Can you work these out from the model? Positions are in its coordinate system, mm. A direction names the side the tool comes from. Coordinates: 2 decimals unless noted, no trailing zeros. Loops run counter-clockwise (first coordinate to the right, second up) from the corner with the lowest first, then second, coordinate; pieces in that order, holes last. Notation, with made-up numbers: M 15,82.25 L 53,82.25 A25 cw 53,119.25 Z; hole C -14.75,35.5 d2. An arc over 180 degrees is marked long. Answer as a JSON object with one key per item and string values. Group by question number.
Item 1: Which directions (+Z, -Z, +X, -X, +Y, -Y) give clear straight access to the entire face, cutting with the end or side of a thin tool? Please do faces 1 (the flat face through (36, 16, 67)), 2 (the flat face through (36, -13.82, 34)).
Item 2: Suppose I cut it at B-B (x = 11). Write out the boundary of the cut face in (y, z).
Item 3: Suppose I cut it at C-C (z = 38). Write out the boundary of the cut face in (x, y), then the cut area to 3 significant figures.
Item 4: Suppose I cut it at D-D (y = -5). Write out the boundary of the cut face in (x, z), then the cut area to 3 significant figures.
Item 5: If I drill on line 1 (Z direction, x = -54, y = 15.5); line 2 (X direction, y = 24.5, z = 38); line 3 (Y direction, x = 38, z = 21), over which ranges is the centre line in solid material (lowest first)?
Item 6: I'm going to push flat-ended pins straight in: pin 1 Ø0.6 at (x, z) = (-71.5, 18.5) entering from +Y; pin 2 Ø1 at (x, z) = (-39.5, 67.5) entering from +Y; pin 3 Ø1.6 at (x, z) = (112.5, 68) entering from +Y. Where does each tip first touch, or does it pass through?
Item 7: Suppose I cut it at A-A (y = 32.5). Write out the boundary of the cut face in (x, z).
Item 8: We'd pull the mould along Z, two halves only. Please class faces 3 (the flat face through (36, 16, 2)), 4 (the flat face through (68, 43.18, 1)), 5 (the flat face through (36, 15, 0)): +Z half, -Z half, draft (parallel to the pull), parting line (faces both ways), or undercut.
```python
from build123d import *

# Parameters (mm, degrees)
ESQUISSE1_W            = 220
ESQUISSE1_H            = 57
BOSS_EXTRU_1_DEPTH     = 69
COQUE1_T               = -2
ESQUISSE2_W            = 42.430934458
ESQUISSE2_H            = 23.81944652
TROU_CABLES_DEPTH      = 10
ESQUISSE4_W            = 39.063130892
ESQUISSE4_H            = 19.851704837
TROU_BORNIER_DEPTH     = 10
ESQUISSE5_W            = 15.700605502
ESQUISSE5_H            = 14.772120087
TROU_RASPBERRY_1_DEPTH = 10
ESQUISSE6_W            = 14.187422576
ESQUISSE6_H            = 17.21673515
TROU_RASPBERRY_2_DEPTH = 10
ESQUISSE7_W            = 14.101040577
ESQUISSE7_H            = 17.33071114
TROU_RASPBERRY_3_DEPTH = 10
ESQUISSE8_W            = 7.498357612
ESQUISSE8_H            = 7.301962728
TROU_RASPBERRY_4_DEPTH = 10
ESQUISSE9_W            = 15.051909722
ESQUISSE9_H            = 7.770311475
TROU_RASPBERRY_5_DEPTH = 10
ESQUISSE10_W           = 8.572607217
ESQUISSE10_H           = 3.212302761
TROU_RASPBERRY_6_DEPTH = 10


with BuildPart() as part:
    # Esquisse1 → Boss.-Extru.1 (new body)
    with BuildSketch(Plane.XY):
        with Locations((37.797752809, 14.679775281)):
            Rectangle(ESQUISSE1_W, ESQUISSE1_H)
    extrude(amount=BOSS_EXTRU_1_DEPTH)

    # Coque1
    coque1_openings = [part.faces().sort_by_distance(p)[0] for p in [
        (37.797752809, 43.179775281, 34.5),
    ]]
    offset(amount=COQUE1_T, openings=coque1_openings, kind=Kind.INTERSECTION)

    # Esquisse2 → Trou cables (cut)
    with BuildSketch(Plane(origin=(0, 0, 0), x_dir=(-1, 0, 0), z_dir=(0, 0, -1))):
        with Locations((45.673767677, 31.270052021)):
            Rectangle(ESQUISSE2_W, ESQUISSE2_H)
    extrude(amount=-TROU_CABLES_DEPTH, mode=Mode.SUBTRACT)

    # Esquisse4 → trou bornier (cut)
    with BuildSketch(Plane.XY.offset(69)):
        with Locations((116.674495492, 33.253922863)):
            Rectangle(ESQUISSE4_W, ESQUISSE4_H)
    extrude(amount=-TROU_BORNIER_DEPTH, mode=Mode.SUBTRACT)

    # Esquisse5 → trou raspberry 1 (cut)
    with BuildSketch(Plane.ZY.offset(72.202247191)):
        with Locations((56.756295127, 35.793715238)):
            Rectangle(ESQUISSE5_W, ESQUISSE5_H)
    extrude(amount=-TROU_RASPBERRY_1_DEPTH, mode=Mode.SUBTRACT)

    # Esquisse6 → trou raspberry 2 (cut)
    with BuildSketch(Plane.ZY.offset(72.202247191)):
        with Locations((37.961253625, 34.571407706)):
            Rectangle(ESQUISSE6_W, ESQUISSE6_H)
    extrude(amount=-TROU_RASPBERRY_2_DEPTH, mode=Mode.SUBTRACT)

    # Esquisse7 → trou raspberry 3 (cut)
    with BuildSketch(Plane.ZY.offset(72.202247191)):
        with Locations((19.999072944, 34.514419711)):
            Rectangle(ESQUISSE7_W, ESQUISSE7_H)
    extrude(amount=-TROU_RASPBERRY_3_DEPTH, mode=Mode.SUBTRACT)

    # Esquisse8 → trou raspberry 4 (cut)
    with BuildSketch(Plane.XY.offset(69)):
        with Locations((-38.723319171, 39.528793917)):
            Rectangle(ESQUISSE8_W, ESQUISSE8_H)
    extrude(amount=-TROU_RASPBERRY_4_DEPTH, mode=Mode.SUBTRACT)

    # Esquisse9 → trou raspberry 5 (cut)
    with BuildSketch(Plane.XY.offset(69)):
        with Locations((-18.817046732, 39.294619544)):
            Rectangle(ESQUISSE9_W, ESQUISSE9_H)
    extrude(amount=-TROU_RASPBERRY_5_DEPTH, mode=Mode.SUBTRACT)

    # Esquisse10 → trou raspberry 6 (cut)
    with BuildSketch(Plane.XY.offset(69)):
        with Locations((0.345482943, 41.573623901)):
            Rectangle(ESQUISSE10_W, ESQUISSE10_H)
    extrude(amount=-TROU_RASPBERRY_6_DEPTH, mode=Mode.SUBTRACT)


solid = part.part
```
From the geometry:
{
 "1": {"face 1": "+Y", "face 2": "+Z, -Z, +X, -X, -Y"},
 "2": {"outline": "M -13.82,0 L 43.18,0 L 43.18,2 L -11.82,2 L -11.82,67 L 43.18,67 L 43.18,69 L -13.82,69 Z"},
 "3": {"outline": "M -72.2,-13.82 L 147.8,-13.82 L 147.8,43.18 L 145.8,43.18 L 145.8,-11.82 L -70.2,-11.82 L -70.2,25.96 L -72.2,25.96 Z", "area": "626 mm2"},
 "4": {"outline": "M -72.2,0 L 147.8,0 L 147.8,69 L -72.2,69 Z; hole M -70.2,2 L 145.8,2 L 145.8,67 L -70.2,67 Z", "area": "1,140 mm2"},
 "5": {"line 1": "0 to 2, 67 to 69", "line 2": "-72.2 to -70.2, 145.8 to 147.8", "line 3": "-13.82 to -11.82"},
 "6": {"pin 1": "y = 25.85", "pin 2": "y = 35.88", "pin 3": "y = 23.33"},
 "7": {"outline": "M -72.2,0 L -66.89,0 L -66.89,2 L -70.2,2 L -70.2,12.95 L -72.2,12.95 Z; M -72.2,27.05 L -70.2,27.05 L -70.2,30.87 L -72.2,30.87 Z; M -72.2,45.05 L -70.2,45.05 L -70.2,48.91 L -72.2,48.91 Z; M -72.2,64.61 L -70.2,64.61 L -70.2,67 L 97.14,67 L 97.14,69 L -72.2,69 Z; M -24.46,0 L 147.8,0 L 147.8,69 L 136.21,69 L 136.21,67 L 145.8,67 L 145.8,2 L -24.46,2 Z"},
 "8": {"face 3": "undercut", "face 4": "draft", "face 5": "-Z half"}
}
